Autodesk Inventor part; units mm, degrees
ref_plane "YZ Plane" through (0, 0, 0) normal (1, 0, 0) x (0, 1, 0)
ref_plane "XZ Plane" through (0, 0, 0) normal (0, 1, 0) x (-1, 0, 0)
ref_plane "XY Plane" through (0, 0, 0) normal (0, 0, 1) x (1, 0, 0)
sketch "Sketch11" plane through (0, 0, 0) normal (0, 0, 1) x (1, 0, 0)
  line L0 (-3.4593, 3.4593) -> (0, 0)
  line L1 (-3.4593, 3.4593) -> (-3.4593, 46.5407)
  line L2 (0, 50) -> (-3.4593, 46.5407)
  line L3 (43.0814, 50) -> (0, 50)
  line L4 (46.5407, 46.5407) -> (43.0814, 50)
  line L5 (46.5407, 3.4593) -> (46.5407, 46.5407)
  line L6 (43.0814, 0) -> (46.5407, 3.4593)
  line L7 (43.0814, 0) -> (0, 0)
extrude "Extrusion8" add sketch "Sketch11" along normal blind 5
sketch "Sketch16" plane through (0, 0, 0) normal (0, 0, -1) x (-1, 0, 0)
  line L0 (-27.0407, 40) -> (-34.0407, 40)
  line L1 (-36.5407, 37.5) -> (-36.5407, 30.5)
  arc A0 (-34.0407, 40) -> (-36.5407, 37.5) centre (-34.0407, 37.5) ccw
  line L2 (-9.0407, 40) -> (-16.0407, 40)
  arc A1 (-6.5407, 37.5) -> (-9.0407, 40) centre (-9.0407, 37.5) ccw
  line L3 (-6.5407, 30.5) -> (-6.5407, 37.5)
  line L4 (-6.5407, 12.5) -> (-6.5407, 19.5)
  arc A2 (-9.0407, 10) -> (-6.5407, 12.5) centre (-9.0407, 12.5) ccw
  line L5 (-16.0407, 10) -> (-9.0407, 10)
  line L6 (-34.0407, 10) -> (-27.0407, 10)
  arc A3 (-36.5407, 12.5) -> (-34.0407, 10) centre (-34.0407, 12.5) ccw
  line L7 (-36.5407, 19.5) -> (-36.5407, 12.5)
  line L8 (0, 50) -> (3.4593, 46.5407)
  line L9 (-43.0814, 0) -> (-46.5407, 3.4593)
  line L10 (-46.5407, 46.5407) -> (-43.0814, 50)
  line L11 (-43.0814, 0) -> (-43.0814, 50)
  line L12 (3.4593, 3.4593) -> (0, 0)
  line L13 (-6.5407, 30.5) -> (-6.5407, 19.5)
  line L14 (-16.0407, 40) -> (-27.0407, 40)
  line L15 (-36.5407, 30.5) -> (-36.5407, 19.5)
  line L16 (-27.0407, 10) -> (-16.0407, 10)
  circle A4 centre (-2.5407, 44) radius 2.5
  circle A5 centre (-40.5407, 6) radius 2.5
  circle A6 centre (-2.5407, 6) radius 2.5
  circle A7 centre (-40.5407, 44) radius 2.5
  line L17 (0, 50) -> (3.4593, 46.5407)
  line L18 (3.4593, 46.5407) -> (3.4593, 3.4593)
  line L19 (0, 0) -> (-43.0814, 0)
  line L20 (3.4593, 3.4593) -> (0, 0)
  line L21 (0, 0) -> (-43.0814, 0)
  line L22 (-43.0814, 0) -> (-46.5407, 3.4593)
  line L23 (-43.0814, 0) -> (-46.5407, 3.4593)
  line L24 (-46.5407, 3.4593) -> (-46.5407, 46.5407)
  line L25 (-46.5407, 3.4593) -> (-46.5407, 46.5407)
  line L26 (-46.5407, 46.5407) -> (-43.0814, 50)
  line L27 (0, 50) -> (-43.0814, 50)
  line L28 (0, 50) -> (-43.0814, 50)
  dimension "d44" = 5
  dimension "d45" = 5
  dimension "d46" = 5
  dimension "d47" = 5
extrude "Extrusion11" add sketch "Sketch16" along normal blind 15
sketch "Sketch18" plane through (0, 0, -15) normal (0, 0, -1) x (-1, 0, 0)
  circle A0 centre (-2.5407, 6) radius 2.5
  circle A1 centre (-2.5407, 6) radius 2.5
  circle A2 centre (-40.5407, 6) radius 2.5
  circle A3 centre (-40.5407, 6) radius 2.5
  circle A4 centre (-40.5407, 44) radius 2.5
  circle A5 centre (-40.5407, 44) radius 2.5
  circle A6 centre (-2.5407, 44) radius 2.5
  circle A7 centre (-2.5407, 44) radius 2.5
  point P0 (0, 0)
extrude "Extrusion12" cut sketch "Sketch18" against normal blind 100
sketch "Sketch19" plane through (0, 0, -15) normal (0, 0, -1) x (-1, 0, 0)
  circle A0 centre (-2.5407, 6) radius 2.5
  circle A1 centre (-2.5407, 6) radius 4.3
  circle A2 centre (-40.5407, 6) radius 2.5
  circle A3 centre (-40.5407, 6) radius 4.3
  circle A4 centre (-2.5407, 44) radius 2.5
  circle A5 centre (-2.5407, 44) radius 4.3
  circle A6 centre (-40.5407, 44) radius 2.5
  circle A7 centre (-40.5407, 44) radius 4.3
  point P0 (0, 0)
  dimension "d54" = 8.6
  dimension "d55" = 8.6
  dimension "d56" = 8.6
  dimension "d57" = 8.6
extrude "Extrusion13" cut sketch "Sketch19" against normal blind 10 contours A0 | A1 | A2 | A3 | A5 | A6 | A7
sketch "Sketch20" plane through (0, 0, -15) normal (0, 0, -1) x (-1, 0, 0)
  line L0 (0, 50) -> (-43.0814, 50)
  line L1 (-43.0814, 50) -> (-46.5407, 46.5407)
  line L2 (-46.5407, 46.5407) -> (-46.5407, 3.4593)
  line L3 (-46.5407, 3.4593) -> (-43.0814, 0)
  line L4 (-43.0814, 0) -> (0, 0)
  line L5 (0, 0) -> (3.4593, 3.4593)
  line L6 (3.4593, 3.4593) -> (3.4593, 46.5407)
  line L7 (3.4593, 46.5407) -> (0, 50)
  circle A0 centre (-2.5407, 44) radius 4.3
  circle A1 centre (-40.5407, 44) radius 4.3
  circle A2 centre (-40.5407, 6) radius 4.3
  circle A3 centre (-2.5407, 6) radius 4.3
  arc A4 (-9.0407, 10) -> (-6.5407, 12.5) centre (-9.0407, 12.5) ccw
  line L8 (-9.0407, 10) -> (-34.0407, 10)
  line L9 (-36.5407, 12.5) -> (-36.5407, 37.5)
  arc A5 (-36.5407, 12.5) -> (-34.0407, 10) centre (-34.0407, 12.5) ccw
  line L10 (-6.5407, 37.5) -> (-6.5407, 12.5)
  arc A6 (-6.5407, 37.5) -> (-9.0407, 40) centre (-9.0407, 37.5) ccw
  line L11 (-34.0407, 40) -> (-9.0407, 40)
  arc A7 (-34.0407, 40) -> (-36.5407, 37.5) centre (-34.0407, 37.5) ccw
extrude "Extrusion14" add sketch "Sketch20" along normal blind 25
sketch "Sketch21" plane through (0, 50, 5) normal (0, 1, 0) x (1, 0, 0)
  line L0 (-1.7593, 45) -> (6.8407, 45)
  circle A0 centre (21.6907, 35) radius 2
  dimension "d63" = 4
extrude "Extrusion15" cut sketch "Sketch21" against normal blind 500
sketch "Sketch22" plane through (0, 50, 5) normal (0, 1, 0) x (1, 0, 0)
  circle A0 centre (21.6907, 35) radius 2
  circle A1 centre (21.6907, 35) radius 3.75
  point P0 (0, 5)
  dimension "d67" = 7.5
extrude "Extrusion16" cut sketch "Sketch22" against normal blind 5 contours A0 | A1
sketch "Sketch23" plane through (0, 0, 5) normal (0, -1, 0) x (1, 0, 0)
  circle A0 centre (21.6907, -35) radius 2
  circle A1 centre (21.6907, -35) radius 3.75
  point P0 (0, -5)
  dimension "d70" = 7.5
extrude "Extrusion17" cut sketch "Sketch23" against normal blind 5
sketch "Sketch25" plane through (0, 0, 5) normal (0, 0, 1) x (1, 0, 0)
  circle A0 centre (2.5407, 6) radius 2.5
  circle A1 centre (40.5407, 44) radius 2.5
  circle A2 centre (2.5407, 44) radius 2.5
  circle A3 centre (40.5407, 6) radius 4.3
  circle A4 centre (21.5407, 25) radius 9
  point P0 (0, 0)
  dimension "d75" = 18
extrude "Extrusion18" cut sketch "Sketch25" against normal blind 20 contours A4
sketch "Sketch26" plane through (0, 0, -40) normal (0, 0, -1) x (-1, 0, 0)
  circle A0 centre (-21.5407, 25) radius 9
  arc A1 (-6.5407, 37.5) -> (-9.0407, 40) centre (-9.0407, 37.5) ccw
  line L0 (-9.0407, 40) -> (-34.0407, 40)
  arc A2 (-34.0407, 40) -> (-36.5407, 37.5) centre (-34.0407, 37.5) ccw
  line L1 (-36.5407, 37.5) -> (-36.5407, 12.5)
  arc A3 (-36.5407, 12.5) -> (-34.0407, 10) centre (-34.0407, 12.5) ccw
  line L2 (-34.0407, 10) -> (-9.0407, 10)
  arc A4 (-9.0407, 10) -> (-6.5407, 12.5) centre (-9.0407, 12.5) ccw
  line L3 (-6.5407, 12.5) -> (-6.5407, 37.5)
  circle A5 centre (-21.5407, 25) radius 9.144
  arc A6 (-6.3007, 37.7) -> (-8.8407, 40.24) centre (-8.8407, 37.7) ccw
  line L4 (-8.8407, 40.24) -> (-34.2407, 40.24)
  arc A7 (-34.2407, 40.24) -> (-36.7807, 37.7) centre (-34.2407, 37.7) ccw
  line L5 (-36.7807, 37.7) -> (-36.7807, 12.3)
  arc A8 (-36.7807, 12.3) -> (-34.2407, 9.76) centre (-34.2407, 12.3) ccw
  line L6 (-34.2407, 9.76) -> (-8.8407, 9.76)
  arc A9 (-8.8407, 9.76) -> (-6.3007, 12.3) centre (-8.8407, 12.3) ccw
  line L7 (-6.3007, 12.3) -> (-6.3007, 37.7)
  point P0 (0, 0)
extrude "Extrusion19" cut sketch "Sketch26" against normal blind 40 contours L7 A9 L6 A8 L5 A7 L4 A6
sketch "Sketch27" plane through (40.5407, 44, -5) normal (0, 0, -1) x (-1, 0, 0)
  circle A0 centre (38, -38) radius 2.5
  circle A1 centre (38, -38) radius 4.3
  circle A2 centre (0, -38) radius 2.5
  circle A3 centre (0, -38) radius 4.3
  circle A4 centre (0, 0) radius 2.5
  circle A5 centre (0, 0) radius 4.3
  circle A6 centre (38, 0) radius 4.3
  circle A7 centre (38, 0) radius 2.5
  point P0 (40.5407, -44)
extrude "Extrusion20" add sketch "Sketch27" along normal blind 2
sketch "Sketch28" plane through (0, 0, -40) normal (0, 0, -1) x (-1, 0, 0)
  arc A0 (-34.2407, 40.24) -> (-36.7807, 37.7) centre (-34.2407, 37.7) ccw
  line L0 (-34.2407, 40.24) -> (-8.8407, 40.24)
  arc A1 (-6.3007, 37.7) -> (-8.8407, 40.24) centre (-8.8407, 37.7) ccw
  line L1 (-6.3007, 37.7) -> (-6.3007, 12.3)
  arc A2 (-8.8407, 9.76) -> (-6.3007, 12.3) centre (-8.8407, 12.3) ccw
  line L2 (-8.8407, 9.76) -> (-34.2407, 9.76)
  arc A3 (-36.7807, 12.3) -> (-34.2407, 9.76) centre (-34.2407, 12.3) ccw
  line L3 (-36.7807, 12.3) -> (-36.7807, 37.7)
  line L4 (-43.0814, 50) -> (-46.5407, 46.5407)
  line L5 (-46.5407, 46.5407) -> (-46.5407, 3.4593)
  line L6 (-46.5407, 3.4593) -> (-43.0814, 0)
  line L7 (-43.0814, 0) -> (0, 0)
  line L8 (0, 0) -> (3.4593, 3.4593)
  line L9 (3.4593, 3.4593) -> (3.4593, 46.5407)
  line L10 (3.4593, 46.5407) -> (0, 50)
  line L11 (0, 50) -> (-43.0814, 50)
  circle A4 centre (-2.5407, 6) radius 4.3
  circle A5 centre (-40.5407, 6) radius 4.3
  circle A6 centre (-40.5407, 44) radius 4.3
  circle A7 centre (-2.5407, 44) radius 4.3
  arc A8 (-34.124, 40.1) -> (-36.6407, 37.5833) centre (-34.124, 37.5833) ccw
  line L12 (-34.124, 40.1) -> (-8.9574, 40.1)
  arc A9 (-6.4407, 37.5833) -> (-8.9574, 40.1) centre (-8.9574, 37.5833) ccw
  line L13 (-6.4407, 37.5833) -> (-6.4407, 12.4167)
  arc A10 (-8.9574, 9.9) -> (-6.4407, 12.4167) centre (-8.9574, 12.4167) ccw
  line L14 (-8.9574, 9.9) -> (-34.124, 9.9)
  arc A11 (-36.6407, 12.4167) -> (-34.124, 9.9) centre (-34.124, 12.4167) ccw
  line L15 (-36.6407, 12.4167) -> (-36.6407, 37.5833)
  circle A12 centre (-21.5407, 25) radius 9
  circle A13 centre (-21.5407, 25) radius 8.9173
extrude "Extrusion21" add sketch "Sketch28" against normal blind 40 contours L0 A1 L1 A2 L2 A3 L3 A0
sketch "Sketch29" plane through (21.6907, 5, -30) normal (0, -1, 0) x (1, 0, 0)
  circle A0 centre (0, 0) radius 2
  circle A1 centre (0, 0) radius 2.05
  point P0 (-21.6907, 30)
  dimension "d86" = 4.1
extrude "Extrusion22" cut sketch "Sketch29" against normal blind 100 contours A0 | A1
sketch "Sketch30" plane through (0, 0, -40) normal (0, 0, -1) x (-1, 0, 0)
  circle A0 centre (-2.5407, 44) radius 2.5
  circle A1 centre (-2.5407, 44) radius 2.55
  circle A2 centre (-2.5407, 6) radius 4.3
  circle A3 centre (-2.5407, 6) radius 2.55
  circle A4 centre (-40.5407, 6) radius 2.5
  circle A5 centre (-40.5407, 6) radius 2.55
  circle A6 centre (-40.5407, 44) radius 2.5
  circle A7 centre (-40.5407, 44) radius 2.55
  point P0 (0, 0)
  dimension "d89" = 5.1
  dimension "d90" = 5.1
  dimension "d91" = 5.1
  dimension "d92" = 5.1
extrude "Extrusion23" cut sketch "Sketch30" against normal blind 100 contours A0 | A1 | A3 | A4 | A6 | A7
sketch "Sketch31" plane through (0, 0, -40) normal (0, 0, -1) x (-1, 0, 0)
  arc A0 (-34.2919, 40.3015) -> (-36.8422, 37.7513) centre (-34.2919, 37.7513) ccw
  line L0 (-34.2919, 40.3015) -> (-8.7894, 40.3015)
  arc A1 (-6.2392, 37.7512) -> (-8.7894, 40.3015) centre (-8.7895, 37.7512) ccw
  line L1 (-6.2392, 37.7512) -> (-6.2392, 12.2487)
  arc A2 (-8.7895, 9.6985) -> (-6.2392, 12.2487) centre (-8.7895, 12.2487) ccw
  line L2 (-8.7895, 9.6985) -> (-34.292, 9.6985)
  arc A3 (-36.8422, 12.2488) -> (-34.292, 9.6985) centre (-34.292, 12.2488) ccw
  line L3 (-36.8422, 12.2488) -> (-36.8422, 37.7513)
  circle A4 centre (-21.5407, 25) radius 9
  circle A5 centre (-21.5407, 25) radius 1
  point P0 (0, 0)
  dimension "d95" = 2
extrude "Extrusion24" cut sketch "Sketch31" against normal blind 40 contours L0 A1 L1 A2 L2 A3 L3 A0 | A4 | A5
Read the model definition and answer for the solid it produces. Units are mm, in the model's axes. A direction names the side the tool comes from. Give positions to 0.01 mm unless a question says otherwise; leave off trailing zeros. Loops run counter-clockwise (first coordinate to the right, second up) from the corner with the lowest first, then second, coordinate; pieces in that order, holes last. Notation, with made-up numbers: (-36, 69.25) - (21, 69.25) arc R30 cw to (21, 102.25) - close; hole circle Ø8 at (-31.5, 80). An arc over 180 degrees is marked (long way). Answer as CSV lines item,"result". Start each with the question number.
1) Find section A-A (y = 6). Write down the section's boundary in (x, z), then the cut area to 3 significant figures.
2) Determine the mould class of faces 1 (the face through (23, 5, -32)), 2 (the face through (3, 3, -7)), 3 (the face through (21, 50, -17)) for opening direction Y: released by +Y, released by -Y, zero draft, split by the parting line, or undercut.
3) Find section B-B (y = 25). Write down the section's boundary in (x, z).
4) Find section C-C (z = 1). Write down the section's boundary in (x, y), then the cut area to 3 significant figures.
5) Find section D-D (x = 3). Write down the section's boundary in (y, z).
6) Which of the six approach directions +Z, -Z, +X, -X, +Y, -Y give full straight-line access (tool end or side, diameter ignored) to faces 4 (the face through (22, 40.302, -20)), 5 (the face through (25.268, 2.465, -28.874)), 6 (the face through (-2, 48, -17))?
7) Straight lines are drawn through the part: L1, parallel to Y at x = 30.5, z = -18; L2, parallel to Y at x = 39.5, z = -11; L3, parallel to X at y = 46, z = 1.5. For each, find the intervals that lie inside material, in ascending order. Write a range as from..to.
8) Each of these flat-tipped pins is pushed along its axis until it touches: pin 1 Ø4 at (x, y) = (40.54, 6) entering from -Z; pin 2 Ø4.5 at (x, y) = (41.5, 7.5) entering from -Z; pin 3 Ø6.5 at (x, z) = (21.69, -30) entering from -Y; pin 4 Ø1.5 at (x, y) = (12.5, 28.5) entering from -Z. Where does it stop, or does it pass through?
Findings below:
1,outline,"(-3.46, -40) - (-1.76, -40) - (-1.76, -7) - (-0.01, -7) - (-0.01, 5) - (-3.46, 5) - close; (5.09, -7) - (6.84, -7) - (6.84, -40) - (36.24, -40) - (36.24, -7) - (38.04, -7) - (38.04, 5) - (5.09, 5) - close; (43.04, -7) - (44.84, -7) - (44.84, -40) - (46.54, -40) - (46.54, 5) - (43.04, 5) - close; hole circle Ø4.1 at (21.69, -30)"
1,area,"1,550 mm^2"
2,face 1,"released by -Y"
2,face 2,"undercut"
2,face 3,"released by +Y"
3,outline,"(-3.46, -40) - (6.24, -40) - (6.24, 0) - (12.54, 0) - (12.54, 5) - (-3.46, 5) - close; (30.54, 0) - (36.84, 0) - (36.84, -40) - (46.54, -40) - (46.54, 5) - (30.54, 5) - close"
4,outline,"(-3.46, 3.46) - (0, 0) - (43.08, 0) - (46.54, 3.46) - (46.54, 46.54) - (43.08, 50) - (0, 50) - (-3.46, 46.54) - close; hole circle Ø5.1 at (2.54, 6); hole circle Ø5.1 at (2.54, 44); hole circle Ø18 at (21.54, 25); hole circle Ø5.1 at (40.54, 44); hole circle Ø5 at (40.54, 6)"
4,area,"2,140 mm^2"
5,outline,"(0, -40) - (1.72, -40) - (1.72, -7) - (3.49, -7) - (3.49, 5) - (0, 5) - close; (8.51, -7) - (10.28, -7) - (10.28, -40) - (39.72, -40) - (39.72, -7) - (41.49, -7) - (41.49, 5) - (8.51, 5) - close; (46.51, -7) - (48.28, -7) - (48.28, -40) - (50, -40) - (50, 5) - (46.51, 5) - close"
6,face 4,"-Z"
6,face 5,"-Y"
6,face 6,"+Z, -Z, -X, +Y"
7,L1,"0..9.7, 40.3..50"
7,L2,"0..1.83, 10.17..39.83, 48.17..50"
7,L3,"-3.46..0.96, 4.12..38.96, 42.12..46.54"
8,pin 1,"through"
8,pin 2,"z = -7"
8,pin 3,"y = 5"
8,pin 4,"z = 0"
